Part print with two shaded views. Sizes in mm from the minimum x, y, z corner. A direction names the side the tool comes from. Give positions to 0.01 mm unless a question says otherwise; leave off trailing zeros. Loops run counter-clockwise (first coordinate to the right, second up) from the corner with the lowest first, then second, coordinate; pieces in that order, holes last. Notation, with made-up numbers: M 65.25,-12 L 94.25,-12 A17 ccw 94.25,-8 Z; hole C 44.25,-14.5 d1. An arc over 180 degrees is marked long. Answer as a JSON object with one key per item and string values. Group by question number.
1. Slice it at C-C (x = 39). List the corners of the cut face in (y, z) (3 decimals).
2. Drop flat-ended pins along their axis: pin 1 Ø20 at (x, z) = (22, 15) entering from -Y; pin 2 Ø1.5 at (x, y) = (18, 13.5) entering from +Z; pin 3 Ø5.5 at (x, z) = (43, 24.5) entering from +Y. Give the stop position or say it passes through.
3. 3-axis set-ups, long thin cutter, end or side, ignore diameter. For the marked faces 4 and 5: which of +Z, -Z, +X, -X, +Y, -Y reach the whole face in a straight line?
4. Mould opens along Z. For the marked faces 1, 2 and 3 say: released by +Z, released by -Z, zero draft, split by the parting line, or undercut.
5. Slice it at B-B (z = 3). List the corners of the cut face in (x, y), then the cut area to 3 significant figures.
6. Drill centre lines: line 1 along Y through (x, z) = (39, 2.85); line 2 along X through (y, z) = (43.5, 12); line 3 along X through (y, z) = (42, 24). Where is each one in solid material? Low to high. Write a range as [from, to].
7. Slice it at D-D (z = 9.5). List the corners of the cut face in (x, y), then the cut area to 3 significant figures.
8. Slice it at A-A (y = 7.5). List the corners of the cut face in (x, z).
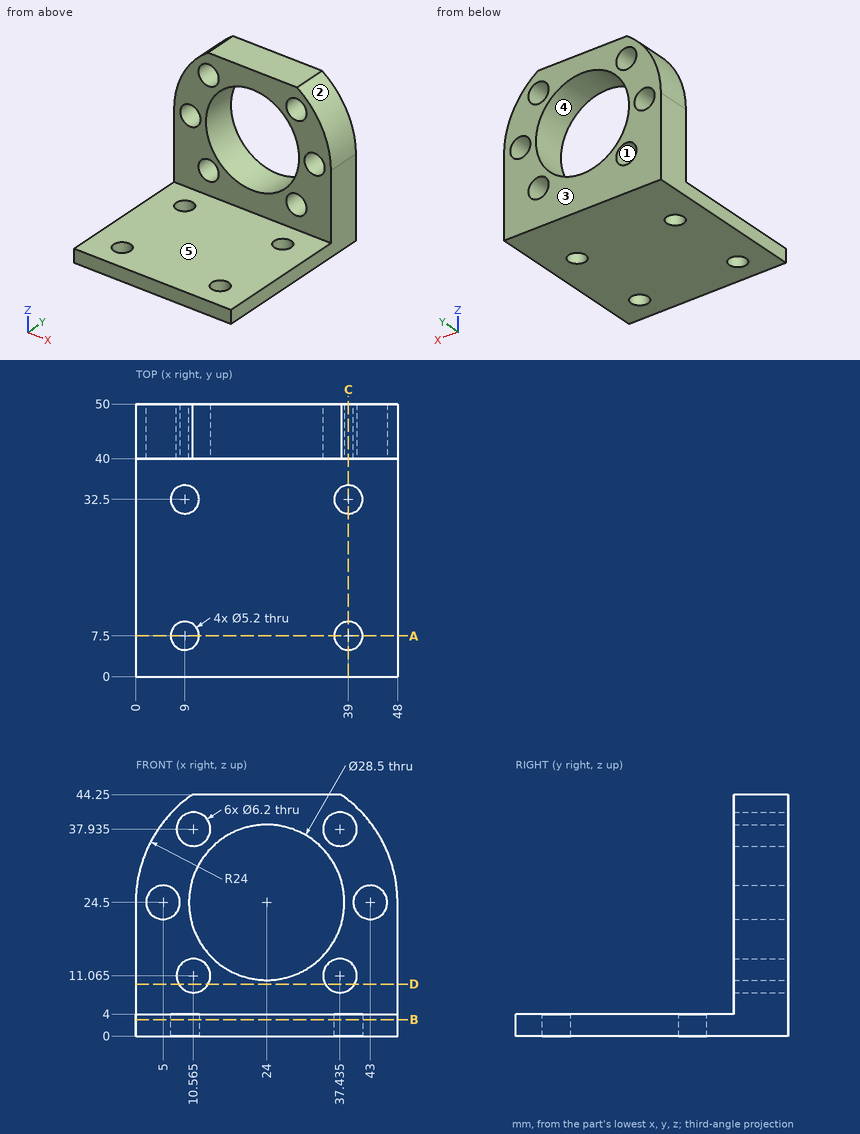
Established:
{
 "1": {"outline": "M 0,0 L 4.9,0 L 4.9,4 L 0,4 Z; M 10.1,0 L 29.9,0 L 29.9,4 L 10.1,4 Z; M 35.1,0 L 50,0 L 50,8.389 L 40,8.389 L 40,4 L 35.1,4 Z; M 40,13.741 L 50,13.741 L 50,35.259 L 40,35.259 Z; M 40,40.611 L 50,40.611 L 50,43.235 L 40,43.235 Z"},
 "2": {"pin 1": "stops at y = 40", "pin 2": "stops at z = 4", "pin 3": "passes through"},
 "3": {"face 4": "+Y, -Y", "face 5": "+Z, +X, -X, -Y"},
 "4": {"face 1": "undercut", "face 2": "released by +Z", "face 3": "zero draft"},
 "5": {"outline": "M 0,0 L 48,0 L 48,50 L 0,50 Z; hole C 9,7.5 d5.2; hole C 9,32.5 d5.2; hole C 39,7.5 d5.2; hole C 39,32.5 d5.2", "area": "2,320 mm^2"},
 "6": {"line 1": "y = [0, 4.9], [10.1, 29.9], [35.1, 50]", "line 2": "x = [0, 7.61], [13.52, 17.16], [30.84, 34.48], [40.39, 48]", "line 3": "x = [0, 1.94], [8.06, 9.76], [38.24, 39.94], [46.06, 48]"},
 "7": {"outline": "M 0,40 L 7.89,40 L 7.89,50 L 0,50 Z; M 13.24,40 L 34.76,40 L 34.76,50 L 13.24,50 Z; M 40.11,40 L 48,40 L 48,50 L 40.11,50 Z", "area": "373 mm^2"},
 "8": {"outline": "M 0,0 L 6.4,0 L 6.4,4 L 0,4 Z; M 11.6,0 L 36.4,0 L 36.4,4 L 11.6,4 Z; M 41.6,0 L 48,0 L 48,4 L 41.6,4 Z"}
}
